Check sheet for the modelled part. Datum: model origin and axes. Units: mm. A direction names the side the tool comes from. Round coordinates to 2 decimals unless told otherwise and drop trailing zeros. Order: outer loops, then holes, each group sorted by start corner. A loop starts at its lowest first (then second) coordinate and runs counter-clockwise, first axis right, second up.
from build123d import *

# Parameters (mm, degrees)
SKETCH1_W           = 20
SKETCH1_H           = 80
BOSS_EXTRUDE1_DEPTH = 30
FILLET1_R           = 2
SKETCH2_R           = 4
CUT_EXTRUDE1_DEPTH  = 10
CUT_EXTRUDE2_START  = -10
SKETCH3_R           = 4
CUT_EXTRUDE2_DEPTH  = 10


with BuildPart() as part:
    # Sketch1 → Boss-Extrude1 (new body)
    with BuildSketch(Plane.XY):
        with Locations((10, 40)):
            Rectangle(SKETCH1_W, SKETCH1_H)
    extrude(amount=BOSS_EXTRUDE1_DEPTH)

    # Fillet1
    fillet1_edges = [part.edges().sort_by_distance(p)[0] for p in [
        (10, 80, 30),
        (20, 40, 30),
        (10, 0, 30),
        (20, 40, 0),
        (10, 80, 0),
        (0, 40, 0),
        (10, 0, 0),
        (20, 0, 15),
        (20, 80, 15),
        (0, 80, 15),
        (0, 0, 15),
        (0, 40, 30),
    ]]
    fillet(fillet1_edges, radius=FILLET1_R)

    # Sketch2 → Cut-Extrude1 (cut)
    with BuildSketch(Plane(origin=(0, 80, 0), x_dir=(1, 0, 0), z_dir=(0, 1, 0))):
        with Locations(Location((10, -15, 0), (0, 0, 270))):
            Circle(SKETCH2_R)
    extrude(amount=-CUT_EXTRUDE1_DEPTH, mode=Mode.SUBTRACT)

    # Sketch3 → Cut-Extrude2 (cut)
    with BuildSketch(Plane.XZ.offset(CUT_EXTRUDE2_START)):
        with Locations(Location((10, 15, 0), (0, 0, 90))):
            Circle(SKETCH3_R)
    extrude(amount=CUT_EXTRUDE2_DEPTH, mode=Mode.SUBTRACT)


solid = part.part
1) Gauge pin test, flat end, axial feed: pin 1 (2.5 mm diameter, centred on x = 8.5, z = 16.5, fed in from +Y). Record the tip position at first contact, or that the pin passes through.
2) Scan lines: line 1 (Z direction, x = 10, y = 7.5); line 2 (X direction, y = 74.5, z = 15); line 3 (Y direction, x = 15.5, z = 1.75). Record each from-to range of solid material in increasing order.
3) Set-up check for faces 5 (the face through (12.4, 5.1, 11.8)), 6 (the face through (10, 75, 11)), 7 (the face through (19.43, 40.53, 29.4)): record each of +Z, -Z, +X, -X, +Y, -Y from which the full face is reachable in a straight line by a thin tool's end or side.
4) Sectioned sample at B-B on x = 10. Record the cut outline in (y, z).
5) Sectioned sample at A-A on z = 15. Record the cut outline in (x, y), and give its area (3 significant figures).
6) Draft check along X on faces 1 (the face through (10, 70, 15)), 2 (the face through (10.11, 79.43, 0.6)), 3 (the face through (10, 10, 15)), 4 (the face through (0.57, 40.53, 29.4)). Enter one of: pulls with the +X half, pulls with the -X half, needs draft (parallel to the pull), parting line crosses it, or undercut.
Values found:
1. pin 1: stops at y = 70
2. line 1: z = 0 to 11, 19 to 30
2. line 2: x = 0 to 6, 14 to 20
2. line 3: y = 0.02 to 79.98
3. face 5: -Y
3. face 6: +Y
3. face 7: +Z, +X, +Y, -Y
4. outline: (0, 2) arc R2 ccw to (2, 0) - (78, 0) arc R2 ccw to (80, 2) - (80, 11) - (70, 11) - (70, 19) - (80, 19) - (80, 28) arc R2 ccw to (78, 30) - (2, 30) arc R2 ccw to (0, 28) - (0, 19) - (10, 19) - (10, 11) - (0, 11) - close
5. outline: (0, 2) arc R2 ccw to (2, 0) - (6, 0) - (6, 10) - (14, 10) - (14, 0) - (18, 0) arc R2 ccw to (20, 2) - (20, 78) arc R2 ccw to (18, 80) - (14, 80) - (14, 70) - (6, 70) - (6, 80) - (2, 80) arc R2 ccw to (0, 78) - close
5. area: 1,440 mm2
6. face 1: undercut
6. face 2: needs draft
6. face 3: undercut
6. face 4: pulls with the -X half
